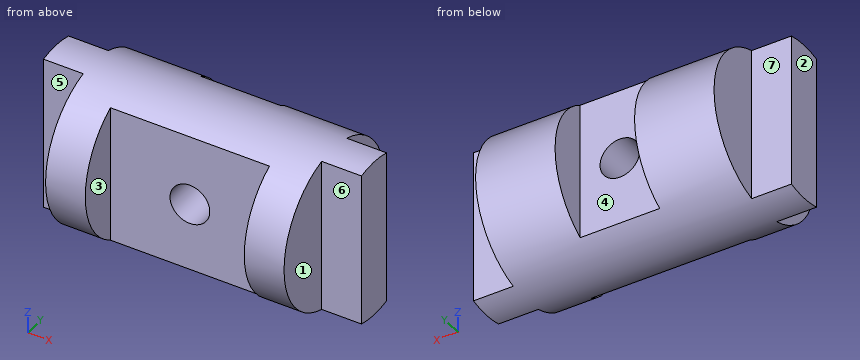
```python
from build123d import *

# Parameters (mm, degrees)
SKETCH1_R                           = 20
BOSS_EXTRUDE1_DEPTH                 = 80
CUT_EXTRUDE1_REACH                  = 86.853
CUT_EXTRUDE1_END_RADIUS             = 20
SKETCH2_W                           = 20
SKETCH2_H                           = 10
SKETCH2_W_2                         = 10
SKETCH2_H_2                         = 15
SKETCH2_W_3                         = 40
CUT_EXTRUDE1_DIRECTION_2_REACH      = 86.853
CUT_EXTRUDE1_DIRECTION_2_END_RADIUS = 20
CUT_EXTRUDE2_REACH                  = 89.75
SKETCH3_R                           = 5


with BuildPart() as part:
    # Sketch1 → Boss-Extrude1 (new body)
    with BuildSketch(Plane(origin=(0, 0, 0), x_dir=(0, 0, -1), z_dir=(1, 0, 0))):
        Circle(SKETCH1_R)
    extrude(amount=BOSS_EXTRUDE1_DEPTH)

    # Cut-Extrude1: up to this cylinder (the profile starts inside it)
    cut_extrude1_end = Plane(origin=(40, 0, 0), z_dir=(-1, 0, 0)) * Cylinder(CUT_EXTRUDE1_END_RADIUS, 284.706, mode=Mode.PRIVATE)
    # Sketch2 → Cut-Extrude1 (cut, up to the surface)
    with BuildSketch(Plane.XY, mode=Mode.PRIVATE) as cut_extrude1_sk1:
        with Locations((40, 15)):
            Rectangle(SKETCH2_W, SKETCH2_H)
    cut_extrude1_tool1 = extrude(cut_extrude1_sk1.sketch, amount=-CUT_EXTRUDE1_REACH, mode=Mode.PRIVATE) & cut_extrude1_end
    add(cut_extrude1_tool1.solids().sort_by_distance((40, 15, 0))[0], mode=Mode.SUBTRACT)
    # Sketch2 → Cut-Extrude1 (cut, up to the surface)
    with BuildSketch(Plane.XY, mode=Mode.PRIVATE) as cut_extrude1_sk2:
        with Locations((5, 12.5)):
            Rectangle(SKETCH2_W_2, SKETCH2_H_2)
    cut_extrude1_tool2 = extrude(cut_extrude1_sk2.sketch, amount=-CUT_EXTRUDE1_REACH, mode=Mode.PRIVATE) & cut_extrude1_end
    add(cut_extrude1_tool2.solids().sort_by_distance((5, 12.5, 0))[0], mode=Mode.SUBTRACT)
    # Sketch2 → Cut-Extrude1 (cut, up to the surface)
    with BuildSketch(Plane.XY, mode=Mode.PRIVATE) as cut_extrude1_sk3:
        with Locations((5, -12.5)):
            Rectangle(SKETCH2_W_2, SKETCH2_H_2)
    cut_extrude1_tool3 = extrude(cut_extrude1_sk3.sketch, amount=-CUT_EXTRUDE1_REACH, mode=Mode.PRIVATE) & cut_extrude1_end
    add(cut_extrude1_tool3.solids().sort_by_distance((5, -12.5, 0))[0], mode=Mode.SUBTRACT)
    # Sketch2 → Cut-Extrude1 (cut, up to the surface)
    with BuildSketch(Plane.XY, mode=Mode.PRIVATE) as cut_extrude1_sk4:
        with Locations((75, 12.5)):
            Rectangle(SKETCH2_W_2, SKETCH2_H_2)
    cut_extrude1_tool4 = extrude(cut_extrude1_sk4.sketch, amount=-CUT_EXTRUDE1_REACH, mode=Mode.PRIVATE) & cut_extrude1_end
    add(cut_extrude1_tool4.solids().sort_by_distance((75, 12.5, 0))[0], mode=Mode.SUBTRACT)
    # Sketch2 → Cut-Extrude1 (cut, up to the surface)
    with BuildSketch(Plane.XY, mode=Mode.PRIVATE) as cut_extrude1_sk5:
        with Locations((75, -12.5)):
            Rectangle(SKETCH2_W_2, SKETCH2_H_2)
    cut_extrude1_tool5 = extrude(cut_extrude1_sk5.sketch, amount=-CUT_EXTRUDE1_REACH, mode=Mode.PRIVATE) & cut_extrude1_end
    add(cut_extrude1_tool5.solids().sort_by_distance((75, -12.5, 0))[0], mode=Mode.SUBTRACT)
    # Sketch2 → Cut-Extrude1 (cut, up to the surface)
    with BuildSketch(Plane.XY, mode=Mode.PRIVATE) as cut_extrude1_sk6:
        with Locations((40, -15)):
            Rectangle(SKETCH2_W_3, SKETCH2_H)
    cut_extrude1_tool6 = extrude(cut_extrude1_sk6.sketch, amount=-CUT_EXTRUDE1_REACH, mode=Mode.PRIVATE) & cut_extrude1_end
    add(cut_extrude1_tool6.solids().sort_by_distance((40, -15, 0))[0], mode=Mode.SUBTRACT)

    # Cut-Extrude1 direction 2: up to this cylinder (the profile starts inside it)
    cut_extrude1_direction_2_end = Plane(origin=(40, 0, 0), z_dir=(-1, 0, 0)) * Cylinder(CUT_EXTRUDE1_DIRECTION_2_END_RADIUS, 284.706, mode=Mode.PRIVATE)
    # Sketch2 → Cut-Extrude1 direction 2 (cut, up to the surface)
    with BuildSketch(Plane.XY, mode=Mode.PRIVATE) as cut_extrude1_direction_2_sk1:
        with Locations((40, 15)):
            Rectangle(SKETCH2_W, SKETCH2_H)
    cut_extrude1_direction_2_tool1 = extrude(cut_extrude1_direction_2_sk1.sketch, amount=CUT_EXTRUDE1_DIRECTION_2_REACH, mode=Mode.PRIVATE) & cut_extrude1_direction_2_end
    add(cut_extrude1_direction_2_tool1.solids().sort_by_distance((40, 15, 0))[0], mode=Mode.SUBTRACT)
    # Sketch2 → Cut-Extrude1 direction 2 (cut, up to the surface)
    with BuildSketch(Plane.XY, mode=Mode.PRIVATE) as cut_extrude1_direction_2_sk2:
        with Locations((5, 12.5)):
            Rectangle(SKETCH2_W_2, SKETCH2_H_2)
    cut_extrude1_direction_2_tool2 = extrude(cut_extrude1_direction_2_sk2.sketch, amount=CUT_EXTRUDE1_DIRECTION_2_REACH, mode=Mode.PRIVATE) & cut_extrude1_direction_2_end
    add(cut_extrude1_direction_2_tool2.solids().sort_by_distance((5, 12.5, 0))[0], mode=Mode.SUBTRACT)
    # Sketch2 → Cut-Extrude1 direction 2 (cut, up to the surface)
    with BuildSketch(Plane.XY, mode=Mode.PRIVATE) as cut_extrude1_direction_2_sk3:
        with Locations((5, -12.5)):
            Rectangle(SKETCH2_W_2, SKETCH2_H_2)
    cut_extrude1_direction_2_tool3 = extrude(cut_extrude1_direction_2_sk3.sketch, amount=CUT_EXTRUDE1_DIRECTION_2_REACH, mode=Mode.PRIVATE) & cut_extrude1_direction_2_end
    add(cut_extrude1_direction_2_tool3.solids().sort_by_distance((5, -12.5, 0))[0], mode=Mode.SUBTRACT)
    # Sketch2 → Cut-Extrude1 direction 2 (cut, up to the surface)
    with BuildSketch(Plane.XY, mode=Mode.PRIVATE) as cut_extrude1_direction_2_sk4:
        with Locations((75, 12.5)):
            Rectangle(SKETCH2_W_2, SKETCH2_H_2)
    cut_extrude1_direction_2_tool4 = extrude(cut_extrude1_direction_2_sk4.sketch, amount=CUT_EXTRUDE1_DIRECTION_2_REACH, mode=Mode.PRIVATE) & cut_extrude1_direction_2_end
    add(cut_extrude1_direction_2_tool4.solids().sort_by_distance((75, 12.5, 0))[0], mode=Mode.SUBTRACT)
    # Sketch2 → Cut-Extrude1 direction 2 (cut, up to the surface)
    with BuildSketch(Plane.XY, mode=Mode.PRIVATE) as cut_extrude1_direction_2_sk5:
        with Locations((75, -12.5)):
            Rectangle(SKETCH2_W_2, SKETCH2_H_2)
    cut_extrude1_direction_2_tool5 = extrude(cut_extrude1_direction_2_sk5.sketch, amount=CUT_EXTRUDE1_DIRECTION_2_REACH, mode=Mode.PRIVATE) & cut_extrude1_direction_2_end
    add(cut_extrude1_direction_2_tool5.solids().sort_by_distance((75, -12.5, 0))[0], mode=Mode.SUBTRACT)
    # Sketch2 → Cut-Extrude1 direction 2 (cut, up to the surface)
    with BuildSketch(Plane.XY, mode=Mode.PRIVATE) as cut_extrude1_direction_2_sk6:
        with Locations((40, -15)):
            Rectangle(SKETCH2_W_3, SKETCH2_H)
    cut_extrude1_direction_2_tool6 = extrude(cut_extrude1_direction_2_sk6.sketch, amount=CUT_EXTRUDE1_DIRECTION_2_REACH, mode=Mode.PRIVATE) & cut_extrude1_direction_2_end
    add(cut_extrude1_direction_2_tool6.solids().sort_by_distance((40, -15, 0))[0], mode=Mode.SUBTRACT)

    # Sketch3 → Cut-Extrude2 (cut, up to next)
    with BuildSketch(Plane(origin=(0, 10, 0), x_dir=(1, 0, 0), z_dir=(0, 1, 0)), mode=Mode.PRIVATE) as cut_extrude2_sk1:
        with Locations(Location((40, 0.320508076, 0), (0, 0, 180))):
            Circle(SKETCH3_R)
    cut_extrude2_tool1 = extrude(cut_extrude2_sk1.sketch, amount=-CUT_EXTRUDE2_REACH, mode=Mode.PRIVATE) & part.part
    add(cut_extrude2_tool1.solids().sort_by_distance((40, 10, -0.320508))[0], mode=Mode.SUBTRACT)


solid = part.part
```
Can you work these out from the model? Positions are in its coordinate system, mm. Face numbers are marked on the shaded views. A direction names the side the tool comes from. Round coordinates to 2 decimals unless told otherwise and drop trailing zeros. Loops run counter-clockwise (first coordinate to the right, second up) from the corner with the lowest first, then second, coordinate; pieces in that order, holes last. Notation, with made-up numbers: M 47,70.25 L 93,70.25 A11 ccw 93,82.25 Z; hole C 29,1.5 d9. An arc over 180 degrees is marked long. Answer as a JSON object with one key per item and string values. Group by question number.
Q1. Will these pins go through, and if not, where does the flat tip stop? pin 1 (5 mm diameter, centred on x = 73, z = 5.5, fed in from -Y); pin 2 (16 mm diameter, centred on x = 40.5, z = 1.5, fed in from +Y); pin 3 (10.5 mm diameter, centred on x = 37, z = 7.5, fed in from -Y); pin 4 (8 mm diameter, centred on x = 40, z = -0.32, fed in from +Y).
Q2. We'd pull the mould along X, two halves only. Please class the marked faces 1, 2 and 3: +X half, -X half, draft (parallel to the pull), parting line (faces both ways), or undercut.
Q3. Imagine slicing it at C-C, the plane z = -16. Please give me the cut outline in (x, y), then the cut area to 3 significant figures.
Q4. Imagine slicing it at A-A, the plane x = 40. Please give me the cut outline in (y, z), then the cut area to 3 significant figures.
Q5. Please list where these lines run through material, in increasing order: L1, parallel to X at y = 16.5, z = 9.5; L2, parallel to X at y = -10.5, z = -4.5; L3, parallel to Y at x = 45, z = 11.
Q6. On a 3-axis mill with a long thin cutter (end or side, diameter ignored), from which of +Z, -Z, +X, -X, +Y, -Y can I reach the whole of each face in a straight line? I mean the marked faces 4, 5, 6 and 7. Say none if no direction works.
Q7. Imagine slicing it at D-D, the plane x = 52. Please give me the cut outline in (y, z).
Q8. Imagine slicing it at B-B, the plane z = -3.5. Please give me the cut outline in (x, y), then the cut area to 3 significant figures.
Findings:
{
 "1": {"pin 1": "stops at y = -5", "pin 2": "stops at y = 10", "pin 3": "stops at y = -10", "pin 4": "passes through"},
 "2": {"face 1": "+X half", "face 2": "-X half", "face 3": "undercut"},
 "3": {"outline": "M 0,-5 L 10,-5 L 10,-12 L 20,-12 L 20,-10 L 60,-10 L 60,-12 L 70,-12 L 70,-5 L 80,-5 L 80,5 L 70,5 L 70,12 L 50,12 L 50,10 L 30,10 L 30,12 L 10,12 L 10,5 L 0,5 Z", "area": "1,520 mm2"},
 "4": {"outline": "M -10,-17.32 A20 ccw 10,-17.32 L 10,-5.32 L -10,-5.32 Z; M -10,4.68 L 10,4.68 L 10,17.32 A20 ccw -10,17.32 Z", "area": "565 mm2"},
 "5": {"L1": "x = 10 to 30, 50 to 70", "L2": "x = 10 to 20, 60 to 70", "L3": "y = -10 to 10"},
 "6": {"face 4": "+Z, -Z, +Y", "face 5": "+Z, -Z, -X, -Y", "face 6": "+Z, -Z, +X, -Y", "face 7": "+Z, -Z, -X, +Y"},
 "7": {"outline": "M -10,-17.32 A20 ccw long -10,17.32 Z"},
 "8": {"outline": "M 0,-5 L 10,-5 L 10,-19.69 L 20,-19.69 L 20,-10 L 36.14,-10 L 36.14,10 L 30,10 L 30,19.69 L 10,19.69 L 10,5 L 0,5 Z; M 43.86,-10 L 60,-10 L 60,-19.69 L 70,-19.69 L 70,-5 L 80,-5 L 80,5 L 70,5 L 70,19.69 L 50,19.69 L 50,10 L 43.86,10 Z", "area": "1,830 mm2"}
}
